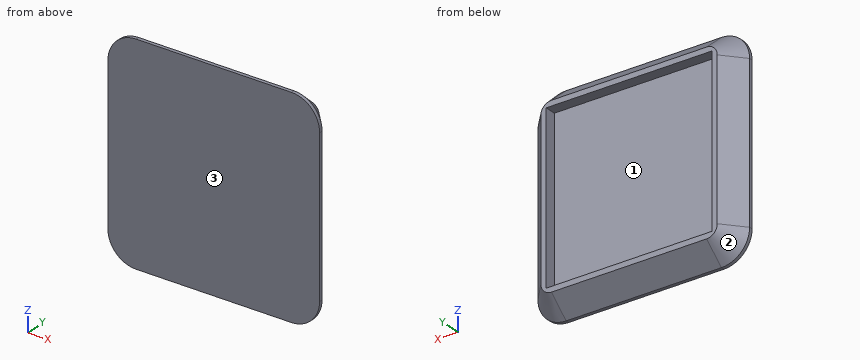
Autodesk Inventor part; units mm, degrees
ref_plane "YZ Plane" through (0, 0, 0) normal (1, 0, 0) x (0, 1, 0)
ref_plane "XZ Plane" through (0, 0, 0) normal (0, 1, 0) x (-1, 0, 0)
ref_plane "XY Plane" through (0, 0, 0) normal (0, 0, 1) x (1, 0, 0)
sketch "Sketch1" plane through (0, 0, 0) normal (0, 1, 0) x (-1, 0, 0)
  line L0 (30, 30) -> (-30, 30)
  line L1 (-30, 30) -> (-30, -30)
  line L2 (-30, -30) -> (30, -30)
  line L3 (30, -30) -> (30, 30)
  point P0 (0, 0)
  point P1 (30, 0)
  point P2 (0, 30)
  dimension "d0" = 60
  dimension "d1" = 60
extrude "Extrusion1" add sketch "Sketch1" along normal blind 0.96
sketch "Sketch2" plane through (0, 0.96, 0) normal (0, 1, 0) x (1, 0, 0)
  line L0 (30, -30) -> (30, 30)
  line L1 (30, 30) -> (-30, 30)
  line L2 (-30, 30) -> (-30, -30)
  line L3 (-30, -30) -> (30, -30)
  line L4 (-30, 0) -> (30, 0)
  line L5 (0, -30) -> (0, 30)
  circle A0 centre (-12.5, -12.5) radius 4.25
  circle A1 centre (-12.5, 12.5) radius 4.25
  circle A2 centre (12.5, 12.5) radius 4.25
  circle A3 centre (12.5, -12.5) radius 4.25
  point P0 (0, 0)
  dimension "d13" = 8.5
  dimension "d14" = 25
  dimension "d15" = 25
extrude "Extrusion2" add sketch "Sketch2" along normal blind 1.92 contours L3 L5 L4 L0 | L4 L5 L1 L0 | L3 L2 L4 L5 | L4 L2 L1 L5 | A0 | A1 | A2 | A3
sketch "Sketch3" plane through (0, 2.88, 0) normal (0, 1, 0) x (1, 0, 0)
  line L0 (-30, 30) -> (-30, -30)
  line L1 (-30, -30) -> (30, -30)
  line L2 (30, -30) -> (30, 30)
  line L3 (30, 30) -> (-30, 30)
  point P0 (0, 0)
extrude "Extrusion3" add sketch "Sketch3" along normal blind 0.64
fillet "Fillet1" radius 8 4 edges at (30, 1.76, 30) (-30, 1.76, 30) (-30, 1.76, -30) (30, 1.76, -30)
ref_plane "Arbeitsebene2" through (27.6569, 3.52, -27.6569) normal (-0.7071, 0, -0.7071) x (0, -1, 0)
sketch "Skizze7" plane through (0, 3.52, 0) normal (0, 1, 0) x (1, 0, 0)
  line L0 (-22, -30) -> (22, -30)
  arc A0 (22, -30) -> (30, -22) centre (22, -22) ccw
  line L1 (30, -22) -> (30, 22)
  arc A1 (30, 22) -> (22, 30) centre (22, 22) ccw
  line L2 (22, 30) -> (-22, 30)
  arc A2 (-22, 30) -> (-30, 22) centre (-22, 22) ccw
  line L3 (-30, 22) -> (-30, -22)
  arc A3 (-30, -22) -> (-22, -30) centre (-22, -22) ccw
  line L4 (22, -30) -> (-22, -30)
  line L5 (-30, -22) -> (-30, 22)
  line L6 (-22, 30) -> (22, 30)
  line L7 (30, 22) -> (30, -22)
  arc A4 (22, -30) -> (30, -22) centre (22, -22) ccw
  arc A5 (-30, -22) -> (-22, -30) centre (-22, -22) ccw
  arc A6 (-22, 30) -> (-30, 22) centre (-22, 22) ccw
  arc A7 (30, 22) -> (22, 30) centre (22, 22) ccw
  point P0 (0, 0)
extrude "Extrusion4" add sketch "Skizze7" along normal blind 3.2
sketch "Skizze8" plane through (0, 6.72, 0) normal (0, 1, 0) x (1, 0, 0)
  line L0 (23.5, 23.5) -> (-23.5, 23.5)
  line L1 (-23.5, 23.5) -> (-23.5, -23.5)
  line L2 (-23.5, -23.5) -> (23.5, -23.5)
  line L3 (23.5, -23.5) -> (23.5, 23.5)
  line L4 (23.5, 23.5) -> (-23.5, -23.5) construction
  line L5 (-23.5, 23.5) -> (23.5, -23.5) construction
  point P0 (0, 0)
  dimension "d25" = 47
  dimension "d26" = 47
extrude "Extrusion5" cut sketch "Skizze8" against normal blind 3.2
chamfer "Fasen2" distance 5 distance2 5.76 8 edges at (0, 6.72, -30) (-27.6569, 6.72, -27.6569) (-30, 6.72, 0) (-27.6569, 6.72, 27.6569) (0, 6.72, 30) (27.6569, 6.72, 27.6569) (30, 6.72, 0) (27.6569, 6.72, -27.6569) measured on face at (7.3333, 6.72, -25.6667)
properties part number "IMU_Base_T-Shirt"
Part model, mm, in its own coordinate system. Face numbers are marked on the shaded views. Round coordinates to 2 decimals unless told otherwise and drop trailing zeros. Loops run counter-clockwise (first coordinate to the right, second up) from the corner with the lowest first, then second, coordinate; pieces in that order, holes last. Notation, with made-up numbers: (-33.75, 46.25) -> (15.25, 46.25) arc R14 ccw to (15.25, 52.25) -> close; hole circle Ø5 at (38.25, -21). An arc over 180 degrees is marked (long way). Use one line per item in the form item = value. Start each with the question number.
Item 1: Drill centre lines: line 1 along Y through (x, z) = (19, -13.5); line 2 along Z through (x, y) = (22, 6.5); line 3 along X through (y, z) = (4.25, -14). Where is each one in solid material? Low to high.
Item 2: Drop flat-ended pins along their axis: pin 1 Ø3.5 at (y, z) = (5.5, 7.5) entering from +X; pin 2 Ø6 at (x, z) = (-11, -5.5) entering from -Y; pin 3 Ø4 at (y, z) = (5, -18) entering from -X; pin 4 Ø1 at (y, z) = (4.5, 9.5) entering from +X. Give the stop position or say it passes through.
Item 3: Band-saw the part on A-A (z = 2). List the corners of the cut face in (x, y), plus the area to 3 significant figures.
Item 4: Band-saw the part on C-C (y = 5.5). List the corners of the cut face in (x, z).
Item 5: Band-saw the part on D-D (y = 2.25). List the corners of the cut face in (x, z), plus the area to 3 significant figures.
Item 6: Band-saw the part on B-B (x = -7). List the corners of the cut face in (y, z), plus the area to 3 significant figures.
Item 7: Two-plate mould, pull along Z, no slides. Class the marked faces 1, 2 and 3: released by +Z, released by -Z, zero draft, split by the parting line, or undercut.
Data:
q1.line_1 = 0 to 3.52
q1.line_2 = -25.19 to -23.5, 23.5 to 25.19
q1.line_3 = -27.14 to -23.5, 23.5 to 27.14
q2.pin_1 = 27.58
q2.pin_2 = 0
q2.pin_3 = -28.23
q2.pin_4 = 27.36
q3.outline = (-30, 0) -> (30, 0) -> (30, 0.96) -> (25, 6.72) -> (23.5, 6.72) -> (23.5, 3.52) -> (-23.5, 3.52) -> (-23.5, 6.72) -> (-25, 6.72) -> (-30, 0.96) -> close
q3.area = 224 mm^2
q4.outline = (-26.06, -22) arc R4.06 ccw to (-22, -26.06) -> (22, -26.06) arc R4.06 ccw to (26.06, -22) -> (26.06, 22) arc R4.06 ccw to (22, 26.06) -> (-22, 26.06) arc R4.06 ccw to (-26.06, 22) -> close; hole (-23.5, -23.5) -> (23.5, -23.5) -> (23.5, 23.5) -> (-23.5, 23.5) -> close
q5.outline = (-28.88, -22) arc R6.88 ccw to (-22, -28.88) -> (22, -28.88) arc R6.88 ccw to (28.88, -22) -> (28.88, 22) arc R6.88 ccw to (22, 28.88) -> (-22, 28.88) arc R6.88 ccw to (-28.88, 22) -> close
q5.area = 3,300 mm^2
q6.outline = (0, -30) -> (0.96, -30) -> (6.72, -25) -> (6.72, -23.5) -> (3.52, -23.5) -> (3.52, 23.5) -> (6.72, 23.5) -> (6.72, 25) -> (0.96, 30) -> (0, 30) -> close
q6.area = 224 mm^2
q7.face_1 = undercut
q7.face_2 = released by -Z
q7.face_3 = zero draft
